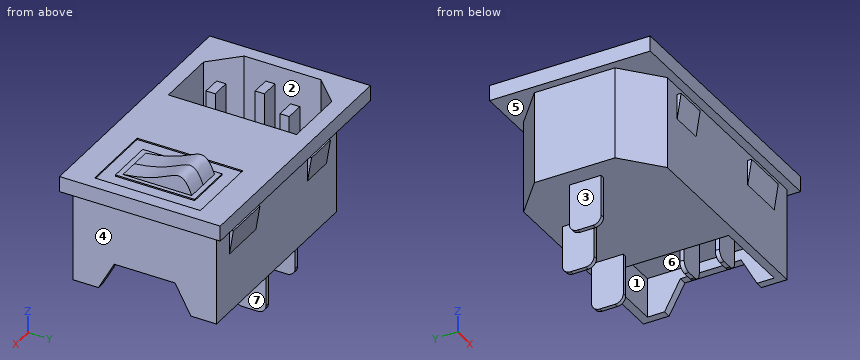
from build123d import *

# Parameters (mm, degrees)
SKETCH1_W           = 50.292
SKETCH1_H           = 30.8864
BOSS_EXTRUDE1_DEPTH = 2.9718
SKETCH2_W           = 47.0916
SKETCH2_H           = 27.6225
BOSS_EXTRUDE2_DEPTH = 17.78
CUT_EXTRUDE1_DEPTH  = 17.78
SKETCH4_W           = 15.24
SKETCH4_H           = 24.384
CUT_EXTRUDE2_DEPTH  = 7.62
CUT_EXTRUDE3_REACH  = 62.341
SKETCH6_W           = 0.8128
SKETCH6_H           = 6.096
BOSS_EXTRUDE3_DEPTH = 9.398
SKETCH7_W           = 5.08
SKETCH7_H           = 0.8128
BOSS_EXTRUDE4_DEPTH = 7.62
FILLET1_R           = 1.5875
CUT_EXTRUDE4_DEPTH  = 19.05
SKETCH9_W           = 3.556
SKETCH9_H           = 1.778
BOSS_EXTRUDE5_DEPTH = 18.415
SKETCH10_W          = 14.224
SKETCH10_H          = 20.32
SKETCH10_W_2        = 9.144
SKETCH10_H_2        = 15.24
CUT_EXTRUDE5_DEPTH  = 0.254
BOSS_EXTRUDE6_START = -9.652
BOSS_EXTRUDE6_DEPTH = 3.81
BOSS_EXTRUDE7_START = -4.318
BOSS_EXTRUDE7_DEPTH = 8.89
BOSS_EXTRUDE8_START = -30.48
BOSS_EXTRUDE8_DEPTH = 6.35


with BuildPart() as part:
    # Sketch1 → Boss-Extrude1 (new body)
    with BuildSketch(Plane.XY):
        with Locations((25.146, 15.4432)):
            Rectangle(SKETCH1_W, SKETCH1_H)
    extrude(amount=BOSS_EXTRUDE1_DEPTH)

    # Sketch2 → Boss-Extrude2 (add)
    with BuildSketch(Plane(origin=(0, 0, 0), x_dir=(-1, 0, 0), z_dir=(0, 0, -1))):
        with Locations((-25.146, 15.4432)):
            Rectangle(SKETCH2_W, SKETCH2_H)
    extrude(amount=BOSS_EXTRUDE2_DEPTH)

    # Sketch3 → Cut-Extrude1 (cut)
    with BuildSketch(Plane(origin=(0, 0, -17.78), x_dir=(-1, 0, 0), z_dir=(0, 0, -1))):
        Polygon((-8.5598, 29.25445), (-1.6002, 23.1902), (-1.6002, 29.25445), align=None)
        Polygon((-1.6002, 1.63195), (-1.6002, 7.6962), (-8.5598, 1.63195), align=None)
    extrude(amount=-CUT_EXTRUDE1_DEPTH, mode=Mode.SUBTRACT)

    # Sketch4 → Cut-Extrude2 (cut)
    with BuildSketch(Plane(origin=(0, 0, -17.78), x_dir=(-1, 0, 0), z_dir=(0, 0, -1))):
        with Locations((-39.5478, 15.4432)):
            Rectangle(SKETCH4_W, SKETCH4_H)
    extrude(amount=-CUT_EXTRUDE2_DEPTH, mode=Mode.SUBTRACT)

    # Sketch5 → Cut-Extrude3 (cut, up to next)
    with BuildSketch(Plane(origin=(48.6918, 0, 0), x_dir=(0, 0, -1), z_dir=(1, 0, 0)), mode=Mode.PRIVATE) as cut_extrude3_sk1:
        Polygon((17.78, 24.3332), (17.78, 6.5532), (12.192, 9.6012), (12.192, 21.2852), align=None)
    cut_extrude3_tool1 = extrude(cut_extrude3_sk1.sketch, amount=-CUT_EXTRUDE3_REACH, mode=Mode.PRIVATE) & part.part
    add(cut_extrude3_tool1.solids().sort_by_distance((48.6918, 15.4432, -15.17869))[0], mode=Mode.SUBTRACT)

    # Sketch6 → Boss-Extrude3 (add)
    with BuildSketch(Plane(origin=(0, 0, -17.78), x_dir=(-1, 0, 0), z_dir=(0, 0, -1))):
        with Locations((-5.5626, 15.4432)):
            Rectangle(SKETCH6_W, SKETCH6_H)
        with Locations((-16.1798, 22.90445)):
            Rectangle(SKETCH6_W, SKETCH6_H)
        with Locations((-28.6258, 24.42845)):
            Rectangle(SKETCH6_W, SKETCH6_H)
    extrude(amount=BOSS_EXTRUDE3_DEPTH)

    # Sketch7 → Boss-Extrude4 (add)
    with BuildSketch(Plane(origin=(0, 0, -10.16), x_dir=(-1, 0, 0), z_dir=(0, 0, -1))):
        with Locations((-39.5478, 8.33755)):
            Rectangle(SKETCH7_W, SKETCH7_H)
        with Locations((-39.5478, 15.14475)):
            Rectangle(SKETCH7_W, SKETCH7_H)
    extrude(amount=BOSS_EXTRUDE4_DEPTH)

    # Fillet1
    fillet1_edges = [part.edges().sort_by_distance(p)[0] for p in [
        (42.0878, 8.33755, -17.78),
        (37.0078, 8.33755, -17.78),
        (42.0878, 15.14475, -17.78),
        (37.0078, 15.14475, -17.78),
        (5.5626, 12.3952, -27.178),
        (5.5626, 18.4912, -27.178),
        (16.1798, 19.85645, -27.178),
        (16.1798, 25.95245, -27.178),
        (28.6258, 21.38045, -27.178),
        (28.6258, 27.47645, -27.178),
    ]]
    fillet(fillet1_edges, radius=FILLET1_R)

    # Sketch8 → Cut-Extrude4 (cut)
    with BuildSketch(Plane.XY.offset(2.9718)):
        Polygon((19.304, 27.7622), (19.304, 3.1242), (7.493, 3.1242), (2.54, 8.0772), (2.54, 15.4432), (2.54, 22.8092), (7.493, 27.7622), align=None)
    extrude(amount=-CUT_EXTRUDE4_DEPTH, mode=Mode.SUBTRACT)

    # Sketch9 → Boss-Extrude5 (add)
    with BuildSketch(Plane.XY.offset(-16.0782)):
        with Locations((12.446, 22.5552)):
            Rectangle(SKETCH9_W, SKETCH9_H)
        with Locations((8.382, 15.4432)):
            Rectangle(SKETCH9_W, SKETCH9_H)
        with Locations((12.446, 8.3312)):
            Rectangle(SKETCH9_W, SKETCH9_H)
    extrude(amount=BOSS_EXTRUDE5_DEPTH)

    # Sketch10 → Cut-Extrude5 (cut)
    with BuildSketch(Plane.XY.offset(2.9718)):
        with Locations((40.64, 15.4432)):
            Rectangle(SKETCH10_W, SKETCH10_H)
        with Locations((40.64, 15.4432)):
            Rectangle(SKETCH10_W_2, SKETCH10_H_2, mode=Mode.SUBTRACT)
    extrude(amount=-CUT_EXTRUDE5_DEPTH, mode=Mode.SUBTRACT)

    # Sketch11 → Boss-Extrude6 (add, symmetric)
    with BuildSketch(Plane(origin=(50.292, 0, 0), x_dir=(0, 0, -1), z_dir=(1, 0, 0)).offset(BOSS_EXTRUDE6_START)):
        with BuildLine():
            Line((-2.9718, 15.4432), (-2.9718, 22.0472))
            add(Edge.make_bspline(
                [(-2.9718, 8.8392), (-3.553872131, 15.290477118), (-8.392581533, 20.316911693), (-3.884219092, 21.66276478), (-2.9718, 22.0472)],
                knots=[0, 0, 0, 0, 0.486211791, 1, 1, 1, 1], degree=3))
            Line((-2.9718, 8.8392), (-2.9718, 15.4432))
        make_face()
    extrude(amount=BOSS_EXTRUDE6_DEPTH, both=True)

    # Sketch12 → Boss-Extrude7 (add)
    with BuildSketch(Plane(origin=(48.6918, 0, 0), x_dir=(0, 0, -1), z_dir=(1, 0, 0)).offset(BOSS_EXTRUDE7_START)):
        Polygon((1.524, 29.25445), (1.524, 30.01645), (6.35, 29.25445), align=None)
        Polygon((1.524, 1.63195), (1.524, 0.86995), (6.35, 1.63195), align=None)
    extrude(amount=-BOSS_EXTRUDE7_DEPTH)

    # Sketch12<2> → Boss-Extrude8 (add)
    with BuildSketch(Plane(origin=(48.6918, 0, 0), x_dir=(0, 0, -1), z_dir=(1, 0, 0)).offset(BOSS_EXTRUDE8_START)):
        Polygon((1.524, 29.25445), (1.524, 30.01645), (6.35, 29.25445), align=None)
        Polygon((1.524, 1.63195), (1.524, 0.86995), (6.35, 1.63195), align=None)
    extrude(amount=-BOSS_EXTRUDE8_DEPTH)


solid = part.part
Check sheet for the modelled part. Datum: model origin and axes. Units: mm. Face numbers are marked on the shaded views. A direction names the side the tool comes from. Give positions to 0.01 mm unless a question says otherwise; leave off trailing zeros. Loops run counter-clockwise (first coordinate to the right, second up) from the corner with the lowest first, then second, coordinate; pieces in that order, holes last. Notation, with made-up numbers: M 69,87.5 L 124,87.5 A15 cw 124,100.5 Z; hole C 69.5,46 d9. An arc over 180 degrees is marked long. Answer as a JSON object with one key per item and string values. Group by question number.
Q1. Material ranges on line 1 along X through (y, z) = (11.5, -12); line 2 along X through (y, z) = (22.5, -2); line 3 along X through (y, z) = (12.5, -15), recorded low to high. Write a range as [from, to].
Q2. Cross-section at B-B on x = 20. Record the cut outline in (y, z).
Q3. Go/stop test with flat-tipped pins: P1, Ø3, axis at y = 8.5, z = -0.5, coming from the +X side; P2, Ø2, axis at y = 8.5, z = -10, coming from the +X side; P3, Ø1.5, axis at x = 24.5, z = -8.5, coming from the -Y side; P4, Ø2, axis at x = 15.5, z = -17.5, coming from the +Y side. Record where each tip stops, or that it passes through.
Q4. Cross-section at C-C on z = -13. Give the number of separate pieces and of enclosed holes in the cut face, then the cut area to 3 significant figures.
Q5. Cross-section at A-A on z = -23.5. Record the cut outline in (x, y), then the cut area to 3 significant figures.
Q6. Release check for a two-part mould opening along X. For the marked faces 5, 6 and 7 record: released by +X, released by -X, zero draft, split by the parting line, or undercut.
Q7. Access from +Z, -Z, +X, -X, +Y, -Y to the whole of each face (thin tool, end or side, straight path). Record for the marked faces 1, 2, 3 and 4.
Evaluation:
{
 "1": {"line 1": "x = [1.6, 2.54], [19.3, 31.93], [47.17, 48.69]", "line 2": "x = [1.6, 2.54], [10.67, 14.22], [19.3, 48.69]", "line 3": "x = [1.6, 2.54], [19.3, 31.93]"},
 "2": {"outline": "M 0,0 L 1.63,0 L 1.63,-17.78 L 29.25,-17.78 L 29.25,0 L 30.89,0 L 30.89,2.97 L 0,2.97 Z"},
 "3": {"P1": "stops at x = 50.29", "P2": "stops at x = 48.69", "P3": "stops at y = 1.63", "P4": "stops at y = 29.25"},
 "4": {"separate pieces": "6", "enclosed holes": "1", "area": "507 mm2"},
 "5": {"outline": "M 5.16,12.4 L 5.97,12.4 L 5.97,18.49 L 5.16,18.49 Z; M 15.77,19.86 L 16.59,19.86 L 16.59,25.95 L 15.77,25.95 Z; M 28.22,21.38 L 29.03,21.38 L 29.03,27.48 L 28.22,27.48 Z", "area": "14.9 mm2"},
 "6": {"face 5": "zero draft", "face 6": "undercut", "face 7": "released by +X"},
 "7": {"face 1": "-Z", "face 2": "+Z", "face 3": "-Z, -X, +Y, -Y", "face 4": "-Z, +X, +Y, -Y"}
}
